The listing builds one solid part. Answer for the finished solid, in the listing's coordinates (mm). A direction names the side the tool comes from. Coordinates: 2 decimals unless noted, no trailing zeros. Order: outer loops, then holes, each group sorted by start corner. A loop starts at its lowest first (then second) coordinate and runs counter-clockwise, first axis right, second up. Notation, with made-up numbers: (58.5, 83.25) -> (93.5, 83.25) arc R31 ccw to (93.5, 109.25) -> close; hole circle Ø11 at (51.5, -8). An arc over 180 degrees is marked (long way). Return JSON: item names as keys, results as strings.
Autodesk Fusion 360 part; units mm, degrees
sketch "Sketch1" plane through (0, 0, 0) normal (0, 1, 0) x (1, 0, 0)
  line L0 (41.5, 24.75) -> (-41.5, 24.75)
  line L1 (-41.5, 24.75) -> (-41.5, -24.75)
  line L2 (-41.5, -24.75) -> (41.5, -24.75)
  line L3 (41.5, -24.75) -> (41.5, 24.75)
  line L4 (41.5, 24.75) -> (-41.5, -24.75) construction
  line L5 (-41.5, 24.75) -> (41.5, -24.75) construction
  line L6 (6, 26.75) -> (-6, 26.75)
  line L7 (-6, 26.75) -> (-6, 22.75)
  line L8 (-6, 22.75) -> (6, 22.75)
  line L9 (6, 22.75) -> (6, 26.75)
  line L10 (6, 26.75) -> (-6, 22.75) construction
  line L11 (-6, 26.75) -> (6, 22.75) construction
  line L12 (6, -26.75) -> (-6, -26.75)
  line L13 (-6, -26.75) -> (-6, -22.75)
  line L14 (-6, -22.75) -> (6, -22.75)
  line L15 (6, -22.75) -> (6, -26.75)
  point P0 (0, 24.75)
  dimension "d1" = 83
  dimension "d2" = 49.5
  dimension "d3" = 12
  dimension "d4" = 4
extrude "Extrude1" add sketch "Sketch1" along normal blind 1.6 contours L0 L1 L2 L3 L7 L8 L9 L13 L14 L15
fillet "Fillet1" radius 1 4 edges at (6, 0.8, 22.75) (-6, 0.8, 22.75) (6, 0.8, -22.75) (-6, 0.8, -22.75)
fillet "Fillet2" radius 1 4 edges at (-41.5, 0.8, -24.75) (-41.5, 0.8, 24.75) (41.5, 0.8, 24.75) (41.5, 0.8, -24.75)
sketch "Sketch2" plane through (0, 1.6, 0) normal (0, 1, 0) x (-1, 0, 0)
  arc A0 (-41.5, -23.75) -> (-40.5, -24.75) centre (-40.5, -23.75) ccw
  line L0 (-40.5, -24.75) -> (-6, -24.75)
  line L1 (-6, -24.75) -> (-6, -23.75)
  arc A1 (-5, -22.75) -> (-6, -23.75) centre (-5, -23.75) ccw
  line L2 (-5, -22.75) -> (5, -22.75)
  arc A2 (6, -23.75) -> (5, -22.75) centre (5, -23.75) ccw
  line L3 (6, -23.75) -> (6, -24.75)
  line L4 (6, -24.75) -> (40.5, -24.75)
  arc A3 (40.5, -24.75) -> (41.5, -23.75) centre (40.5, -23.75) ccw
  line L5 (41.5, -23.75) -> (41.5, 23.75)
  arc A4 (41.5, 23.75) -> (40.5, 24.75) centre (40.5, 23.75) ccw
  line L6 (40.5, 24.75) -> (6, 24.75)
  line L7 (6, 24.75) -> (6, 23.75)
  arc A5 (5, 22.75) -> (6, 23.75) centre (5, 23.75) ccw
  line L8 (5, 22.75) -> (-5, 22.75)
  arc A6 (-6, 23.75) -> (-5, 22.75) centre (-5, 23.75) ccw
  line L9 (-6, 23.75) -> (-6, 24.75)
  line L10 (-6, 24.75) -> (-40.5, 24.75)
  arc A7 (-40.5, 24.75) -> (-41.5, 23.75) centre (-40.5, 23.75) ccw
  line L11 (-41.5, 23.75) -> (-41.5, -23.75)
  circle A8 centre (25, 18.5) radius 1.5
  circle A9 centre (25, -18.5) radius 1.5
  circle A10 centre (-25, -18.5) radius 1.5
  circle A11 centre (-25, 18.5) radius 1.5
  dimension "d11" = 50
  dimension "d12" = 37
  dimension "d13" = 3
  dimension "d14" = 3
  dimension "d15" = 3
  dimension "d16" = 3
extrude "Extrude2" cut sketch "Sketch2" against normal blind 6 contours A8 | A9 | A10 | A11
sketch "Sketch3" plane through (0, 1.6, 0) normal (0, 1, 0) x (-1, 0, 0)
  circle A0 centre (25, 18.5) radius 1.5
  circle A1 centre (-25, 18.5) radius 1.5
  circle A2 centre (25, -18.5) radius 1.5
  circle A3 centre (-25, -18.5) radius 1.5
  arc A4 (-41.5, -23.75) -> (-40.5, -24.75) centre (-40.5, -23.75) ccw
  line L0 (-40.5, -24.75) -> (-6, -24.75)
  line L1 (-6, -24.75) -> (-6, -23.75)
  arc A5 (-5, -22.75) -> (-6, -23.75) centre (-5, -23.75) ccw
  line L2 (-5, -22.75) -> (5, -22.75)
  arc A6 (6, -23.75) -> (5, -22.75) centre (5, -23.75) ccw
  line L3 (6, -23.75) -> (6, -24.75)
  line L4 (6, -24.75) -> (40.5, -24.75)
  arc A7 (40.5, -24.75) -> (41.5, -23.75) centre (40.5, -23.75) ccw
  line L5 (41.5, -23.75) -> (41.5, 23.75)
  arc A8 (41.5, 23.75) -> (40.5, 24.75) centre (40.5, 23.75) ccw
  line L6 (40.5, 24.75) -> (6, 24.75)
  line L7 (6, 24.75) -> (6, 23.75)
  arc A9 (5, 22.75) -> (6, 23.75) centre (5, 23.75) ccw
  line L8 (5, 22.75) -> (-5, 22.75)
  arc A10 (-6, 23.75) -> (-5, 22.75) centre (-5, 23.75) ccw
  line L9 (-6, 23.75) -> (-6, 24.75)
  line L10 (-6, 24.75) -> (-40.5, 24.75)
  arc A11 (-40.5, 24.75) -> (-41.5, 23.75) centre (-40.5, 23.75) ccw
  line L11 (-41.5, 23.75) -> (-41.5, -23.75)
  circle A12 centre (37.75, 20.3) radius 1
  circle A13 centre (37.75, -20.3) radius 1
  circle A14 centre (-37.75, 20.3) radius 1
  circle A15 centre (-37.75, -20.3) radius 1
  dimension "d19" = 75.5
  dimension "d20" = 40.6
  dimension "d21" = 2
  dimension "d22" = 2
  dimension "d23" = 2
  dimension "d24" = 2
extrude "Extrude3" cut sketch "Sketch3" against normal blind 2 contours A12 | A13 | A14 | A15
sketch "Sketch4" plane through (0, 1.6, 0) normal (0, 1, 0) x (-1, 0, 0)
  circle A0 centre (37.75, 20.3) radius 1
  circle A1 centre (37.75, -20.3) radius 1
  circle A2 centre (-37.75, 20.3) radius 1
  circle A3 centre (-37.75, -20.3) radius 1
  circle A4 centre (25, 18.5) radius 1.5
  circle A5 centre (-25, 18.5) radius 1.5
  circle A6 centre (25, -18.5) radius 1.5
  circle A7 centre (-25, -18.5) radius 1.5
  arc A8 (-41.5, -23.75) -> (-40.5, -24.75) centre (-40.5, -23.75) ccw
  line L0 (-40.5, -24.75) -> (-6, -24.75)
  line L1 (-6, -24.75) -> (-6, -23.75)
  arc A9 (-5, -22.75) -> (-6, -23.75) centre (-5, -23.75) ccw
  line L2 (-5, -22.75) -> (5, -22.75)
  arc A10 (6, -23.75) -> (5, -22.75) centre (5, -23.75) ccw
  line L3 (6, -23.75) -> (6, -24.75)
  line L4 (6, -24.75) -> (40.5, -24.75)
  arc A11 (40.5, -24.75) -> (41.5, -23.75) centre (40.5, -23.75) ccw
  line L5 (41.5, -23.75) -> (41.5, 23.75)
  arc A12 (41.5, 23.75) -> (40.5, 24.75) centre (40.5, 23.75) ccw
  line L6 (40.5, 24.75) -> (6, 24.75)
  line L7 (6, 24.75) -> (6, 23.75)
  arc A13 (5, 22.75) -> (6, 23.75) centre (5, 23.75) ccw
  line L8 (5, 22.75) -> (-5, 22.75)
  arc A14 (-6, 23.75) -> (-5, 22.75) centre (-5, 23.75) ccw
  line L9 (-6, 23.75) -> (-6, 24.75)
  line L10 (-6, 24.75) -> (-40.5, 24.75)
  arc A15 (-40.5, 24.75) -> (-41.5, 23.75) centre (-40.5, 23.75) ccw
  line L11 (-41.5, 23.75) -> (-41.5, -23.75)
Item 1: The part is cut by section B-B on x = -37.75. Determine the outline of the cut face in (y, z).
Answer list:
{"outline": "(0, -24.75) -> (1.6, -24.75) -> (1.6, -21.3) -> (0, -21.3) -> close; (0, -19.3) -> (1.6, -19.3) -> (1.6, 19.3) -> (0, 19.3) -> close; (0, 21.3) -> (1.6, 21.3) -> (1.6, 24.75) -> (0, 24.75) -> close"}
Item 2: Which of the six approach directions +Z, -Z, +X, -X, +Y, -Y give full straight-line access (tool end or side, diameter ignored) to faces 5 (the cylindrical face through (26.11, 0.81, 19.51)), 6 (the flat face through (0, 1, 22.75)), 7 (the flat face through (0, 1, -22.75))?
Answer list:
{"face 5": "+Y, -Y", "face 6": "+Z, +Y, -Y", "face 7": "-Z, +Y, -Y"}
Item 3: Flat-ended cylindrical pins translate along their axes: pin 1 (0.8 mm diameter, centred on x = 0, y = 1, fed in from +Z); pin 2 (0.5 mm diameter, centred on y = 0.5, z = -24.5, fed in from +X). Find the tip coordinate at first contact, or state that the pin passes through.
Answer list:
{"pin 1": "z = 22.75", "pin 2": "x = 41.37"}
Item 4: The part is cut by section A-A on z = 18.5. Determine the outline of the cut face in (x, y).
Answer list:
{"outline": "(-41.5, 0) -> (-26.5, 0) -> (-26.5, 1.6) -> (-41.5, 1.6) -> close; (-23.5, 0) -> (23.5, 0) -> (23.5, 1.6) -> (-23.5, 1.6) -> close; (26.5, 0) -> (41.5, 0) -> (41.5, 1.6) -> (26.5, 1.6) -> close"}
Item 5: Determine the mould class of faces 1 (the cylindrical face through (37.29, 0.81, -21.19)), 2 (the flat face through (-23, 1, -24.75)), 3 (the flat face through (-41.5, 1, 0)), 4 (the cylindrical face through (26.11, 0.81, -17.49)) for opening direction X: pulls with the +X half, pulls with the -X half, needs draft (parallel to the pull), parting line crosses it, or undercut.
Answer list:
{"face 1": "undercut", "face 2": "needs draft", "face 3": "pulls with the -X half", "face 4": "undercut"}
Item 6: The part is cut by section C-C on y = 0.95. Count the separate pieces of the cut face and the enclosed holes in it, plus the area to 3 significant figures.
Answer list:
{"separate pieces": "1", "enclosed holes": "8", "area": "4,020 mm2"}
Item 7: Find the intervals of material crossed by probe 1 along Z at (x, y) = (-25, 0.95); probe 2 along Z at (x, y) = (37.75, 0.85); probe 3 along X at (y, z) = (0.8, 19), in increasing order.
Answer list:
{"probe 1": "-24.75 to -20, -17 to 17, 20 to 24.75", "probe 2": "-24.75 to -21.3, -19.3 to 19.3, 21.3 to 24.75", "probe 3": "-41.5 to -26.41, -23.59 to 23.59, 26.41 to 41.5"}
Item 8: The part is cut by section D-D on x = 0.5. Determine the outline of the cut face in (y, z), plus the area to 3 significant figures.
Answer list:
{"outline": "(0, -22.75) -> (1.6, -22.75) -> (1.6, 22.75) -> (0, 22.75) -> close", "area": "72.8 mm2"}
